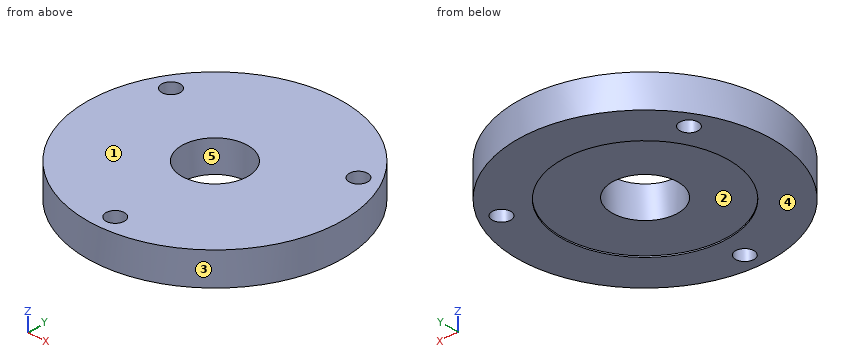
Autodesk Inventor part; units mm, degrees
ref_plane "YZ Plane" through (0, 0, 0) normal (1, 0, 0) x (0, 1, 0)
ref_plane "XZ Plane" through (0, 0, 0) normal (0, 1, 0) x (-1, 0, 0)
ref_plane "XY Plane" through (0, 0, 0) normal (0, 0, 1) x (1, 0, 0)
sketch "Skizze1" plane through (0, 0, 0) normal (0, 1, 0) x (-1, 0, 0)
  line L0 (-3.6106, 0) -> (-3.6106, -12.505)
  line L1 (-38.6, 0) -> (0, 0)
  line L2 (-13.05, -7.505) -> (-13.05, -21.905)
  line L3 (-25.55, -7.505) -> (-25.55, -21.905)
  line L4 (-6.3, -0.4913) -> (-6.3, 0)
  line L5 (-32.3, -0.4913) -> (-6.3, -0.4913)
  line L6 (0, 0) -> (0, 5)
  line L7 (0, 5) -> (-14.3, 5)
  line L8 (-14.3, 5) -> (-14.3, 0.2)
  line L9 (-14.3, 0.2) -> (-6.65, 0.2)
  line L10 (-6.65, 0.2) -> (-6.65, 0)
  line L11 (0, 0) -> (-6.65, 0)
  line L12 (-19.3, -19.905) -> (-19.3, 13.9284)
  dimension "d0" = 5
  dimension "d1" = 12.65
  dimension "d2" = 12.5
  dimension "d3" = 6.25
  dimension "d4" = 0.2
  dimension "d6" = 5
revolve "Umdrehung1" add sketch "Skizze1" angle 360 about axis through (19.3, 0, -19.905) along (0, 0, 1) contours L10 L9 L8 L7 L6 L1
sketch "Skizze2" plane through (19.3, 0, 5) normal (0, 0, 1) x (1, 0, 0)
  circle A0 centre (0, -16.5) radius 1.4
  circle A1 centre (0, 0) radius 19.3
  circle A2 centre (0, 0) radius 12.65
  circle A3 centre (-14.2894, 8.25) radius 1.4
  circle A4 centre (14.2894, 8.25) radius 1.4
  point P0 (-19.3, 0)
extrude "Extrusion1" cut sketch "Skizze2" against normal through all contours A0 | A3 | A4
equation "\"d3\" = 0.5 * d2"
properties part number "50_ETL_Lid_v0"
For this review, take the finished solid that the model builds, in its own axes (mm). Face numbers are marked on the shaded views. A direction names the side the tool comes from. Round coordinates to 2 decimals unless told otherwise and drop trailing zeros. Order: outer loops, then holes, each group sorted by start corner. A loop starts at its lowest first (then second) coordinate and runs counter-clockwise, first axis right, second up. Notation, with made-up numbers: (-21.5, 40) -> (8.5, 40) arc R25 ccw to (8.5, 65) -> close; hole circle Ø2 at (-7.75, 89). An arc over 180 degrees is marked (long way). Put each result on its own line as item: value.
Q1. Insertion check: pin 1 Ø1.7 at (x, y) = (33.59, 8.25) entering from -Z; pin 2 Ø1 at (y, z) = (-11.5, 4.5) entering from +X; pin 3 Ø1 at (x, z) = (21, 2) entering from -Y; pin 4 Ø16 at (x, y) = (19.3, 0) entering from -Z. Each pin has a flat end and moves straight along its axis. Give the tip position at first contact, or say it passes through.
Check result:
pin 1: through
pin 2: x = 35.16
pin 3: y = -19.26
pin 4: z = 0.2
Q2. Add section B-B on x = 19.3. Write out the cut boundary in (y, z), plus the area to 3 significant figures.
Check result:
outline: (-19.3, 0) -> (-17.9, 0) -> (-17.9, 5) -> (-19.3, 5) -> close; (-15.1, 0) -> (-12.65, 0) -> (-12.65, 0.2) -> (-5, 0.2) -> (-5, 5) -> (-15.1, 5) -> close; (5, 0.2) -> (12.65, 0.2) -> (12.65, 0) -> (19.3, 0) -> (19.3, 5) -> (5, 5) -> close
area: 126 mm2
Q3. For probe 1 along Y at (x, z) = (19.3, 2.2); probe 2 along Y at (x, z) = (19.3, 0.1); probe 3 along X at (y, z) = (0, 0.15), list the stretches that pass through material, from the lowest coordinate up. Write a range as [from, to].
Check result:
probe 1: [-19.3, -17.9], [-15.1, -5], [5, 19.3]
probe 2: [-19.3, -17.9], [-15.1, -12.65], [12.65, 19.3]
probe 3: [0, 6.65], [31.95, 38.6]
Q4. Add section D-D on y = 8.25. Write out the cut boundary in (x, z), plus the area to 3 significant figures.
Check result:
outline: (1.85, 0) -> (3.61, 0) -> (3.61, 5) -> (1.85, 5) -> close; (6.41, 0) -> (9.71, 0) -> (9.71, 0.2) -> (28.89, 0.2) -> (28.89, 0) -> (32.19, 0) -> (32.19, 5) -> (6.41, 5) -> close; (34.99, 0) -> (36.75, 0) -> (36.75, 5) -> (34.99, 5) -> close
area: 143 mm2
Q5. Add section A-A on y = 0. Write out the cut boundary in (x, z).
Check result:
outline: (0, 0) -> (6.65, 0) -> (6.65, 0.2) -> (14.3, 0.2) -> (14.3, 5) -> (0, 5) -> close; (24.3, 0.2) -> (31.95, 0.2) -> (31.95, 0) -> (38.6, 0) -> (38.6, 5) -> (24.3, 5) -> close
Q6. Add section C-C on x = 33. Write out the cut boundary in (y, z).
Check result:
outline: (-13.59, 0) -> (6.98, 0) -> (6.98, 5) -> (-13.59, 5) -> close; (9.52, 0) -> (13.59, 0) -> (13.59, 5) -> (9.52, 5) -> close
Q7. Mouldability with a two-part tool opening along X and no side actions: class the marked faces 3, 4 and 5 as pulls with the +X half, pulls with the -X half, needs draft (parallel to the pull), parting line crosses it, or undercut.
Check result:
face 3: parting line crosses it
face 4: needs draft
face 5: undercut
Q8. Machinability: for the marked faces 1 and 2, which of the approach directions +Z, -Z, +X, -X, +Y, -Y give a long, thin tool a straight path to every point of the face, cutting with its end or side? Answer none if there is none.
Check result:
face 1: +Z, +X, -X, +Y, -Y
face 2: -Z
